Could you check a few things on this model? Use its own coordinates, in mm. Face numbers are marked on the shaded views. Round coordinates to 2 decimals unless told otherwise and drop trailing zeros. Write each loop counter-clockwise with the first axis right and the second up, starting at its lowest first coordinate (ties: lowest second). Pieces come first, ordered by that corner, then holes. Notation, with made-up numbers: (4, 76) - (39, 76) arc R12 ccw to (39, 81) - close; hole circle Ø7 at (3, -10). An arc over 180 degrees is marked (long way). Write each question's results on one line, items separated by ' | '. Start each with the question number.
(1) Please list where these lines run through material, in increasing order: line 1 (Z direction, x = -2.6, y = 0); line 2 (Z direction, x = -2.2, y = 0.2); line 3 (Y direction, x = -2.55, z = 0.9). Write a range as [from, to].
(2) Imagine slicing it at A-A on x = -0.8. Write out the boundary of the cut face in (y, z) (1 decimal), then the cut area to 3 significant figures.
(3) Thinking about a two-plate mould opening in Z: for the marked faces 1, 2 and 3, which applies, +Z half, -Z half, draft (parallel to the pull), parting line (faces both ways), or undercut?
(4) For P1, Ø1, axis at x = -1, y = 0.5, coming from the -Z side, with a flat end and sliding along its axis, tell me the tip position at first contact or that it passes through.
```python
from build123d import *

# Parameters (mm, degrees)
CUT_EXTRUDE1_REACH          = 9.645
CIRPATTERN1_COUNT           = 4
DRAFT1_ANGLE                = 5
CHAMFER1_SIZE               = 0.120396
CHAMFER1_SIZE2              = 0.110273872
SKETCH8_W                   = 2.54
SKETCH8_H                   = 5.08
SCREW_SHORTENING_DEPTH      = 6.221219053
SCREW_SHORTENING_DEPTH_BACK = 6.221219053


with BuildPart() as part:
    # Sketch2 → Revolve1 (revolve)
    with BuildSketch(Plane.XY, mode=Mode.PRIVATE) as revolve1_sk:
        Polygon((-3.175, 0), (3.175, 0), (3.175, 1.5875), (-1.8288, 1.5875), (-1.8288, 1.839666194), (-3.175, 3.0099), align=None)
    revolve(revolve1_sk.sketch.rotate(Axis((-3.175, 0, 0), (1, 0, 0)), 180), axis=Axis((-3.175, 0, 0), (1, 0, 0)))

    # Cut-Extrude1: up to this cone (the profile starts inside it)
    cut_extrude1_end = Plane(origin=(-3.175, 0, 0), z_dir=(-1, 0, 0)).offset(-1.933209747) * Cone(1e-06, 11.960277355, 13.758724211, align=(Align.CENTER, Align.CENTER, Align.MIN), mode=Mode.PRIVATE)
    # Sketch3 → Cut-Extrude1 (cut, up to the surface)
    with BuildSketch(Plane.ZY.offset(3.175), mode=Mode.PRIVATE) as cut_extrude1_sk1:
        with BuildLine():
            Line((0, 0), (2.0066, 0))
            ThreePointArc((2.0066, 0), (1.996438885, 0.201681283), (1.966058447, 0.40132))
            Line((1.966058447, 0.40132), (1.183689224, 0.40132))
            Line((1.183689224, 0.40132), (0.63047064, 0.63047064))
            Line((0.63047064, 0.63047064), (0.40132, 1.183689224))
            Line((0.40132, 1.183689224), (0.40132, 1.966058447))
            ThreePointArc((0.40132, 1.966058447), (0.201681283, 1.996438885), (0, 2.0066))
            Line((0, 2.0066), (0, 0))
        make_face()
    cut_extrude1_tool1 = extrude(cut_extrude1_sk1.sketch, amount=-CUT_EXTRUDE1_REACH, mode=Mode.PRIVATE) & cut_extrude1_end
    cut_extrude1 = cut_extrude1_tool1.solids().sort_by_distance((-3.175, 1.0033, 0.028378))[0]
    add(cut_extrude1, mode=Mode.SUBTRACT)

    # CirPattern1: Cut-Extrude1 ×4 about axis
    cirpattern1_axis = Axis((0, 0, 0), (1, 0, 0))
    for i in range(1, CIRPATTERN1_COUNT):
        add(cut_extrude1.rotate(cirpattern1_axis, i * 360 / CIRPATTERN1_COUNT), mode=Mode.SUBTRACT)

    # Draft1
    draft1_faces = [part.faces().sort_by_distance(p)[0] for p in [
        (-3.009498029, 0.40132, -1.333367825),
        (-2.803736683, 0.526902447, -0.880506376),
        (-2.803736683, 0.880506376, -0.526902447),
        (-3.009498029, 1.333367825, -0.40132),
        (-3.009498029, 1.333367825, 0.40132),
        (-2.803736683, 0.880506376, 0.526902447),
        (-2.803736683, 0.526902447, 0.880506376),
        (-3.009498029, 0.40132, 1.333367825),
        (-3.009498029, -0.40132, 1.333367825),
        (-2.803736683, -0.526902447, 0.880506376),
        (-2.803736683, -0.880506376, 0.526902447),
        (-3.009498029, -1.333367825, 0.40132),
        (-3.009498029, -1.333367825, -0.40132),
        (-2.803736683, -0.880506376, -0.526902447),
        (-2.803736683, -0.526902447, -0.880506376),
        (-3.009498029, -0.40132, -1.333367825),
    ]]
    draft(draft1_faces, Plane(origin=(-3.175, 0, 0), x_dir=(0, -1, 0), z_dir=(-1, 0, 0)), DRAFT1_ANGLE)

    # Chamfer1
    chamfer1_edges = [part.edges().sort_by_distance(p)[0] for p in [
        (-3.175, 3.0099, 0),
    ]]
    chamfer1_side = [part.faces().sort_by_distance(p)[0] for p in [
        (-2.5019, 2.424783097, 0),
    ]]
    chamfer(chamfer1_edges, length=CHAMFER1_SIZE, length2=CHAMFER1_SIZE2, reference=chamfer1_side[0])

    # Sketch8 → Screw Shortening (cut, two sides)
    with BuildSketch(Plane.XY) as screw_shortening_sk:
        with Locations((2.6162, 0)):
            Rectangle(SKETCH8_W, SKETCH8_H)
    extrude(amount=SCREW_SHORTENING_DEPTH, mode=Mode.SUBTRACT)
    extrude(screw_shortening_sk.sketch, amount=-SCREW_SHORTENING_DEPTH_BACK, mode=Mode.SUBTRACT)


solid = part.part
```
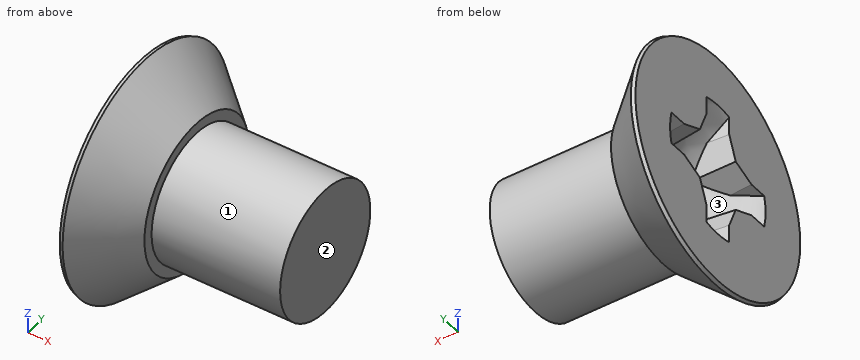
Response:
1) line 1: [-2.51, -1.18], [1.18, 2.51] | line 2: [-2.15, -0.81], [0.81, 2.15] | line 3: [-2.3, -0.46], [0.46, 2.3]
2) outline: circle Ø3.2 at (0, 0) | area: 7.92 mm²
3) face 1: parting line | face 2: draft | face 3: undercut
4) P1: z = -1.59
